Could you check a few things on this model? Use its own coordinates, in mm. Face numbers are marked on the shaded views. Give positions to 0.01 mm unless a question says otherwise; leave off trailing zeros. Write each loop counter-clockwise with the first axis right and the second up, starting at its lowest first coordinate (ties: lowest second). Pieces come first, ordered by that corner, then holes. Notation, with made-up numbers: M 43.5,-38.75 L 54.5,-38.75 A16 cw 54.5,-33.75 Z; hole C -10.75,52 d10. An arc over 180 degrees is marked long. Use one line per item in the form item = value.
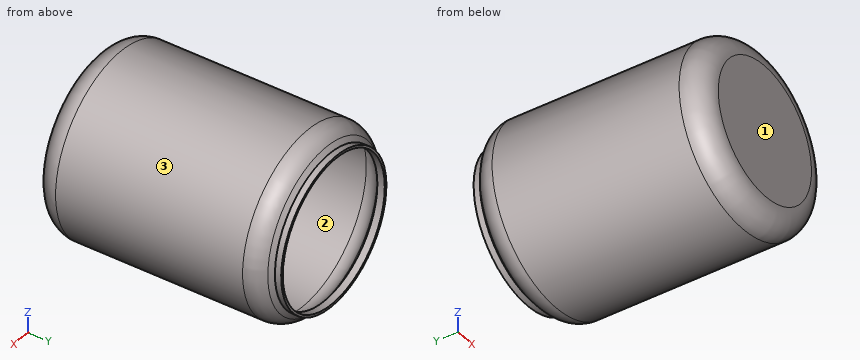
from build123d import *


with BuildPart() as part:
    # Sketch1 → Revolve1 (revolve)
    with BuildSketch(Plane.XY, mode=Mode.PRIVATE) as revolve1_sk:
        with BuildLine():
            Line((39, 90.931199499), (39, 10))
            ThreePointArc((39, 10), (36.071067812, 2.928932188), (29, 0))
            Line((29, 0), (0, 0))
            Line((0, 0), (0, 1))
            Line((0, 1), (29, 1))
            ThreePointArc((29, 1), (35.363961031, 3.636038969), (38, 10))
            Line((38, 10), (38, 90.931199499))
            ThreePointArc((38, 90.931199499), (37.027631255, 95.000245632), (34.320636349, 98.190044369))
            Line((34.320636349, 98.190044369), (31.752687074, 100.072316893))
            Line((31.752687074, 100.072316893), (31.752687074, 103.288460274))
            Line((31.752687074, 103.288460274), (32.752687074, 103.288460274))
            Line((32.752687074, 103.288460274), (32.752687074, 100.579196943))
            Line((32.752687074, 100.579196943), (34.911818166, 98.996582688))
            ThreePointArc((34.911818166, 98.996582688), (37.919590284, 95.452361869), (39, 90.931199499))
        make_face()
    revolve(revolve1_sk.sketch.rotate(Axis((0, 85.763888889, 0), (0, -1, 0)), 90), axis=Axis((0, 85.763888889, 0), (0, -1, 0)))


solid = part.part
1) I want a section at D-D, the plane y = 7. Please give me the cut outline in (x, z).
Checked values:
outline = C 0,0 d77.08; hole C 0,0 d74.97
2) I want a section at B-B, the plane x = 0. Please give me the cut outline in (y, z).
Checked values:
outline = M 0,-29 A10 ccw 10,-39 L 90.93,-39 A10 ccw 99,-34.91 L 100.58,-32.75 L 103.29,-32.75 L 103.29,-31.75 L 100.07,-31.75 L 98.19,-34.32 A9 cw 90.93,-38 L 10,-38 A9 cw 1,-29 L 1,29 A9 cw 10,38 L 90.93,38 A9 cw 98.19,34.32 L 100.07,31.75 L 103.29,31.75 L 103.29,32.75 L 100.58,32.75 L 99,34.91 A10 ccw 90.93,39 L 10,39 A10 ccw 0,29 Z
3) Thinking about a two-plate mould opening in X: for the marked faces 1, 2 and 3, which applies, released by +X, released by -X, zero draft, split by the parting line, or undercut?
Checked values:
face_1 = zero draft
face_2 = undercut
face_3 = split by the parting line
4) If I drill on L1, parallel to X at y = 58, z = -0.5; L2, parallel to X at y = 101, z = 0; L3, parallel to Y at x = -20.5, z = 14.5, over which ranges is the centre line in solid material (lowest first)?
Checked values:
L1 = -39 to -38, 38 to 39
L2 = -32.75 to -31.75, 31.75 to 32.75
L3 = 0 to 1
5) I want a section at A-A, the plane y = 89. Please give me the cut outline in (x, z).
Checked values:
outline = C 0,0 d78; hole C 0,0 d76
6) I want a section at C-C, the plane z = 0. Please give me the cut outline in (x, y).
Checked values:
outline = M -39,10 A10 ccw -29,0 L 29,0 A10 ccw 39,10 L 39,90.93 A10 ccw 34.91,99 L 32.75,100.58 L 32.75,103.29 L 31.75,103.29 L 31.75,100.07 L 34.32,98.19 A9 cw 38,90.93 L 38,10 A9 cw 29,1 L -29,1 A9 cw -38,10 L -38,90.93 A9 cw -34.32,98.19 L -31.75,100.07 L -31.75,103.29 L -32.75,103.29 L -32.75,100.58 L -34.91,99 A10 ccw -39,90.93 Z
7) For pin 1 Ø12 at (x, y) = (-16.5, 74) entering from -Z; pin 2 Ø6 at (x, y) = (25.5, 22.5) entering from -Z; pin 3 Ø12 at (y, z) = (61.5, 2.5) entering from +X; pin 4 Ø10 at (x, y) = (3.5, 26.5) entering from +Z, each with a flat end and sliding along its axis, tell me the tip position at first contact or that it passes through.
Checked values:
pin_1 = -37.56
pin_2 = -31.86
pin_3 = 39
pin_4 = 39
